Model file for the job. Use its own axes, mm. A direction names the side the tool comes from. Give positions to 0.01 mm unless a question says otherwise; leave off trailing zeros. Order: outer loops, then holes, each group sorted by start corner. A loop starts at its lowest first (then second) coordinate and runs counter-clockwise, first axis right, second up. Notation, with made-up numbers: M 27,30.25 L 62,30.25 A27 ccw 62,64.25 Z; hole C -7,49 d8. An arc over 180 degrees is marked long. Return JSON: item names as keys, results as strings. Group by question number.
1. Slice it at A-A on y = 0. List the corners of the cut face in (x, z).
2. Wall check: probe 1 along Y at (x, z) = (160, -15.4); probe 2 along Z at (x, y) = (140, 2.5); probe 3 along Y at (x, z) = (67, 6). Give the ranges that are in metal, low to high. Write a range as [from, to].
3. Pin check, flat tips, straight feed: pin 1 (4 mm diameter, centred on x = 95.5, y = 26, fed in from +Z); pin 2 (3 mm diameter, centred on x = 85, z = -3.5, fed in from -Y); pin 3 (1 mm diameter, centred on y = -26.5, z = -6.5, fed in from +X); pin 4 (9 mm diameter, centred on x = 160, y = 0, fed in from +Z). Stop position of each tip, or through.
4. Slice it at C-C on x = 32. List the corners of the cut face in (y, z), then the cut area to 4 significant figures.
5. 3-axis set-ups, long thin cutter, end or side, ignore diameter. For faces 1 (the face through (97, -62, 17.5)), 2 (the face through (90.63, 60.98, 2.71)): which of +Z, -Z, +X, -X, +Y, -Y reach the whole face in a straight line?
6. Slice it at B-B on z = -1.5. List the corners of the cut face in (x, y), then the cut area to 3 significant figures.
7. Slice it at D-D on y = 18.5. List the corners of the cut face in (x, z), then the cut area to 3 significant figures.
8. Two-plate mould, pull along Y, no slides. Class faces 3 (the face through (5.311, -55.446, 0.245)), 4 (the face through (90.411, 65.977, 0.245)), 5 (the face through (5, 1, 3)): released by +Y, released by -Y, zero draft, split by the parting line, or undercut.
from build123d import *

# Parameters (mm, degrees)
BOSS_EXTRUDE1_DEPTH = 17.5
CUT_EXTRUDE1_DEPTH  = 30
SKETCH6_R           = 7.5
CUT_EXTRUDE2_DEPTH  = 10


with BuildPart() as part:
    # Sketch4 → Boss-Extrude1 (new, symmetric)
    with BuildSketch(Plane.XY):
        with BuildLine():
            Line((0, 41.872855029), (0, -41.872855029))
            ThreePointArc((0, -41.872855029), (5.455474373, -55.600810969), (18.845677428, -61.839515726))
            Line((18.845677428, -61.839515726), (160, -70))
            ThreePointArc((160, -70), (230, 0), (160, 70))
            Line((160, 70), (18.845677428, 61.839515726))
            ThreePointArc((18.845677428, 61.839515726), (5.455474373, 55.600810969), (0, 41.872855029))
        make_face()
    extrude(amount=BOSS_EXTRUDE1_DEPTH, both=True)

    # Sketch5 → Cut-Extrude1 (cut)
    with BuildSketch(Plane.XY.offset(17.5)):
        with BuildLine():
            Line((160.141737643, 64.999845465), (19.134258071, 56.847850552))
            ThreePointArc((19.134258071, 56.847850552), (9.09160578, 52.168821984), (5, 41.872855029))
            Line((5, 41.872855029), (5, -41.872855029))
            ThreePointArc((5, -41.872855029), (9.09160578, -52.168821984), (19.134258071, -56.847850552))
            Line((19.134258071, -56.847850552), (160.141737643, -64.999845465))
            ThreePointArc((160.141737643, -64.999845465), (225, 0), (160.141737643, 64.999845465))
        make_face()
    extrude(amount=-CUT_EXTRUDE1_DEPTH, mode=Mode.SUBTRACT)

    # Sketch6 → Cut-Extrude2 (cut)
    with BuildSketch(Plane(origin=(0, 0, -17.5), x_dir=(-1, 0, 0), z_dir=(0, 0, -1))):
        with Locations((-160, 0)):
            Circle(SKETCH6_R)
    extrude(amount=-CUT_EXTRUDE2_DEPTH, mode=Mode.SUBTRACT)


solid = part.part
Result:
{
 "1": {"outline": "M 0,-17.5 L 152.5,-17.5 L 152.5,-12.5 L 5,-12.5 L 5,17.5 L 0,17.5 Z; M 167.5,-17.5 L 230,-17.5 L 230,17.5 L 225,17.5 L 225,-12.5 L 167.5,-12.5 Z"},
 "2": {"probe 1": "y = [-70, -7.5], [7.5, 70]", "probe 2": "z = [-17.5, -12.5]", "probe 3": "y = [-64.62, -59.62], [59.62, 64.62]"},
 "3": {"pin 1": "stops at z = -12.5", "pin 2": "stops at y = -65.75", "pin 3": "stops at x = 224.99", "pin 4": "passes through"},
 "4": {"outline": "M -62.6,-17.5 L 62.6,-17.5 L 62.6,17.5 L 57.59,17.5 L 57.59,-12.5 L -57.59,-12.5 L -57.59,17.5 L -62.6,17.5 Z", "area": "926.5 mm2"},
 "5": {"face 1": "+Z, +X, -X, +Y, -Y", "face 2": "+Z"},
 "6": {"outline": "M 0,-41.87 A20 ccw 18.85,-61.84 L 160,-70 A70 ccw 160,70 L 18.85,61.84 A20 ccw 0,41.87 Z; hole M 5,-41.87 A15 ccw 19.13,-56.85 L 160.14,-65 A65 ccw 160.14,65 L 19.13,56.85 A15 ccw 5,41.87 Z", "area": "3,160 mm2"},
 "7": {"outline": "M 0,-17.5 L 227.51,-17.5 L 227.51,17.5 L 222.31,17.5 L 222.31,-12.5 L 5,-12.5 L 5,17.5 L 0,17.5 Z", "area": "1,440 mm2"},
 "8": {"face 3": "released by -Y", "face 4": "released by +Y", "face 5": "undercut"}
}
